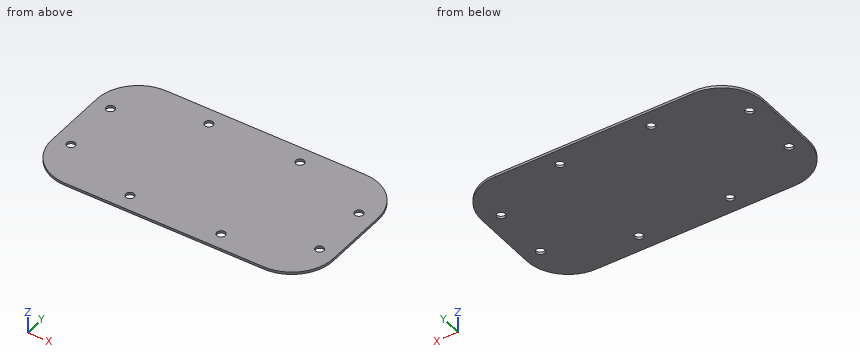
from build123d import *

# Parameters (mm, degrees)
DODANIE_WYCI_GNI_CIE1_DEPTH = 3
OTW_R_GWINTOWANY_M121_D     = 10.2


with BuildPart() as part:
    # Szkic1 → Dodanie-wyciągnięcie1 (new body)
    with BuildSketch(Plane.XY):
        with BuildLine():
            Line((-120, -90), (120, -90))
            ThreePointArc((120, -90), (155.355339059, -75.355339059), (170, -40))
            Line((170, -40), (170, 40))
            ThreePointArc((170, 40), (155.355339059, 75.355339059), (120, 90))
            Line((120, 90), (-120, 90))
            ThreePointArc((-120, 90), (-155.355339059, 75.355339059), (-170, 40))
            Line((-170, 40), (-170, -40))
            ThreePointArc((-170, -40), (-155.355339059, -75.355339059), (-120, -90))
        make_face()
    extrude(amount=DODANIE_WYCI_GNI_CIE1_DEPTH)

    # Otwór gwintowany M121 (through all)
    with Locations(Plane(origin=(0, 0, 0), x_dir=(-1, 0, 0), z_dir=(0, 0, -1))):
        with Locations((55, 70), (-55, 70), (55, -70), (-55, -70), (-150, 35), (-150, -35), (150, -35), (150, 35)):
            Hole(OTW_R_GWINTOWANY_M121_D / 2)


solid = part.part
The model under review builds one solid part; all positions refer to its coordinate system, in mm. Coordinates: 2 decimals unless noted, no trailing zeros. Order: outer loops, then holes, each group sorted by start corner. A loop starts at its lowest first (then second) coordinate and runs counter-clockwise, first axis right, second up. Notation, with made-up numbers: (43, -25) -> (49, -25) arc R20 ccw to (49, 9) -> close; hole circle Ø6 at (-39, -4.5). An arc over 180 degrees is marked (long way). Answer in a Markdown table with one row per item.
(1) Consider section B-B (y = 70). Write out the cut boundary in (x, z), plus the area to 3 significant figures.
Answers:
| item | result |
|---|---|
| outline | (-160, 0) -> (-60.1, 0) -> (-60.1, 3) -> (-160, 3) -> close; (-49.9, 0) -> (49.9, 0) -> (49.9, 3) -> (-49.9, 3) -> close; (60.1, 0) -> (160, 0) -> (160, 3) -> (60.1, 3) -> close |
| area | 899 mm² |
(2) Consider section A-A (x = 150). Write out the cut boundary in (y, z), plus the area to 3 significant figures.
Answers:
| item | result |
|---|---|
| outline | (-80, 0) -> (-40.1, 0) -> (-40.1, 3) -> (-80, 3) -> close; (-29.9, 0) -> (29.9, 0) -> (29.9, 3) -> (-29.9, 3) -> close; (40.1, 0) -> (80, 0) -> (80, 3) -> (40.1, 3) -> close |
| area | 419 mm² |
(3) Wall thickness on line 1 along Y through (x, z) = (55, 1); line 2 along X through (y, z) = (69.5, 1.8); line 3 along X through (y, z) = (37.5, 2.5): over which ranges is each line inside the solid? List them lowest first.
Answers:
| item | result |
|---|---|
| line 1 | -90 to -75.1, -64.9 to 64.9, 75.1 to 90 |
| line 2 | -160.37 to -60.08, -49.92 to 49.92, 60.08 to 160.37 |
| line 3 | -170 to -154.45, -145.55 to 145.55, 154.45 to 170 |
(4) Consider section C-C (z = 0.85). State how many separate pieces and enclosed holes the cut face has, plus the area to 3 significant figures.
Answers:
| item | result |
|---|---|
| separate pieces | 1 |
| enclosed holes | 8 |
| area | 58,400 mm² |
